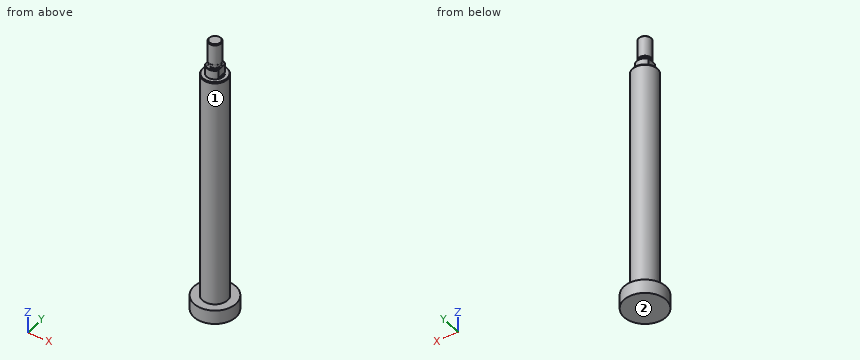
Autodesk Inventor part; units mm, degrees
ref_plane "ANBAU_XY" through (0, 0, -214) normal (0, 0, -1) x (1, 0, 0)
ref_plane "ANBAU_YZ" through (0, 0, -214) normal (1, 0, 0) x (0, -1, 0)
ref_plane "ANBAU_ZX" through (0, 0, -214) normal (0, -1, 0) x (0, 0, -1)
sketch "Sketch_1" plane through (0, 0, 0) normal (1, 0, 0) x (0, 1, 0)
  line L0 (0, -214) -> (0, 29.5)
  line L1 (0, 29.5) -> (7.5, 29.5)
  line L2 (7.5, 29.5) -> (8, 29)
  line L3 (8, 29) -> (8, 20.5)
  line L4 (8, 20.5) -> (11.4226, 20.5)
  line L5 (11.4226, 20.5) -> (12, 19.5)
  line L6 (12, 19.5) -> (12, -200.6667)
  line L7 (12, -200.6667) -> (20, -200.6667)
  line L8 (20, -200.6667) -> (20, -214)
  line L9 (20, -214) -> (0, -214)
  line L10 (0, -214) -> (0, 29.5)
revolve "Revolution1" add sketch "Sketch_1" angle 360 about axis through (0, 0, -214) along (0, 0, -1)
sketch "Sketch_3" plane through (0, 0, 0) normal (0, 1, 0) x (-1, 0, 0)
  line L0 (9.5, 21.5) -> (9.5, 32.5)
  line L1 (9.5, 32.5) -> (-9.5, 32.5)
  line L2 (-9.5, 32.5) -> (-9.5, 21.5)
  line L3 (-9.5, 21.5) -> (-6.5, 21.5)
  line L4 (-6.5, 21.5) -> (-6.5, 29.5)
  line L5 (-6.5, 29.5) -> (6.5, 29.5)
  line L6 (6.5, 29.5) -> (6.5, 21.5)
  line L7 (6.5, 21.5) -> (9.5, 21.5)
extrude "Extrusion1" cut sketch "Sketch_3" along normal mid plane 32
sketch "Sketch_2" plane through (0, 0, 0) normal (1, 0, 0) x (0, 1, 0)
  line L0 (0, 29.5) -> (0, 53.5)
  line L1 (0, 53.5) -> (5.233, 53.5)
  line L2 (5.233, 53.5) -> (6, 52.733)
  line L3 (6, 52.733) -> (6, 33.267)
  line L4 (6, 33.267) -> (5.233, 32.5)
  line L5 (5.233, 32.5) -> (5.233, 30.1)
  arc A0 (5.233, 30.1) -> (5.833, 29.5) centre (5.833, 30.1) ccw
  line L6 (5.833, 29.5) -> (0, 29.5)
  line L7 (0, 29.5) -> (0, 53.5)
revolve "Revolution2" add sketch "Sketch_2" angle 360 about axis through (0, 0, 29.5) along (0, 0, -1)
thread "Thread1"
ref_plane "ANBAU_XY" through (0, 0, -214) normal (0, 0, -1) x (1, 0, 0)
ref_plane "ANBAU_YZ" through (0, 0, -214) normal (1, 0, 0) x (0, -1, 0)
ref_plane "ANBAU_ZX" through (0, 0, -214) normal (0, -1, 0) x (0, 0, -1)
ref_plane "NUT_XY" through (0, 0, 37.5) normal (0, 0, -1) x (1, 0, 0)
ref_plane "NUT_YZ" through (0, 0, 37.5) normal (1, 0, 0) x (0, -1, 0)
ref_plane "NUT_ZX" through (0, 0, 37.5) normal (0, -1, 0) x (0, 0, -1)
properties part number "ESBF-BS-40-100-5P---(KS_0)"
CAD build for the part. Positions are in the model's coordinates, mm. Face numbers are marked on the shaded views. A direction names the side the tool comes from. Coordinates: 2 decimals unless noted, no trailing zeros. Order: outer loops, then holes, each group sorted by start corner. A loop starts at its lowest first (then second) coordinate and runs counter-clockwise, first axis right, second up. Notation, with made-up numbers: (15.5, 34) -> (21.5, 34) arc R26 ccw to (21.5, 57) -> close; hole circle Ø1 at (78.25, 26). An arc over 180 degrees is marked (long way). Use one line per item in the form item = value. Start each with the question number.
1) Band-saw the part on D-D on y = -15.5. Give the cut face in (x, z), then the cut area to 3 significant figures.
2) Drop flat-ended pins along their axis: pin 1 (0.5 mm diameter, centred on x = 7, y = 1.5, fed in from +Z); pin 2 (20 mm diameter, centred on x = -8, y = 3, fed in from +Z); pin 3 (4 mm diameter, centred on y = -3, z = 3.5, fed in from +X); pin 4 (8 mm diameter, centred on y = -10, z = -90.5, fed in from -X). Give the stop position or say it passes through.
3) Band-saw the part on B-B on x = 0. Give the cut face in (y, z).
4) Band-saw the part on C-C on z = -133. Give the cut face in (x, y), then the cut area to 3 significant figures.
5) Tool access for the marked faces 1 and 2: list every direction of +Z, -Z, +X, -X, +Y, -Y with a clear straight run to the whole face (end or side of a thin tool).
6) Drill centre lines: L1, parallel to Z at x = 12.5, y = 0; L2, parallel to Z at x = -2.5, y = 8.5; L3, parallel to X at y = 3, z = -65. Where is each one in solid material? Low to high. Write a range as [from, to].
Entries:
q1.outline = (-12.64, -214) -> (12.64, -214) -> (12.64, -200.67) -> (-12.64, -200.67) -> close
q1.area = 337 mm2
q2.pin_1 = 21.5
q2.pin_2 = 53.5
q2.pin_3 = 11.96
q2.pin_4 = -10.39
q3.outline = (-20, -214) -> (20, -214) -> (20, -200.67) -> (12, -200.67) -> (12, 19.5) -> (11.42, 20.5) -> (8, 20.5) -> (8, 29) -> (7.5, 29.5) -> (5.83, 29.5) arc R0.6 cw to (5.23, 30.1) -> (5.23, 32.5) -> (6, 33.27) -> (6, 52.73) -> (5.23, 53.5) -> (-5.23, 53.5) -> (-6, 52.73) -> (-6, 33.27) -> (-5.23, 32.5) -> (-5.23, 30.1) arc R0.6 cw to (-5.83, 29.5) -> (-7.5, 29.5) -> (-8, 29) -> (-8, 20.5) -> (-11.42, 20.5) -> (-12, 19.5) -> (-12, -200.67) -> (-20, -200.67) -> close
q4.outline = circle Ø24 at (0, 0)
q4.area = 452 mm2
q5.face_1 = +Z
q5.face_2 = -Z, +X, -X, +Y, -Y
q6.L1 = [-214, -200.67]
q6.L2 = [-214, 20.5]
q6.L3 = [-11.62, 11.62]
